Source: CAD feature listing. Evaluate the final solid. Frame: model axes, mm. A direction names the side the tool comes from. Give positions to 0.01 mm unless a question says otherwise; leave off trailing zeros. Order: outer loops, then holes, each group sorted by start corner. A loop starts at its lowest first (then second) coordinate and runs counter-clockwise, first axis right, second up. Notation, with made-up numbers: M 10,-26.75 L 31,-26.75 A15 ccw 31,-0.75 Z; hole C -28.5,89 d3. An arc over 180 degrees is marked long. Answer as a JSON object with one key per item and string values. Group by question number.
1. Section query D-D (y = 0.35). Count the separate pieces of the cut face and the enclosed holes in it, plus the area to 3 significant figures.
2. Section query C-C (z = 5.5). Output: boundary loops of the cut face in (x, y), plus the area to 3 significant figures.
3. Material intervals for L1, parallel to X at y = 1.4, z = 5.5; L2, parallel to X at y = 0.85, z = 5; L3, parallel to X at y = 1.65, z = 3.5, sorted ascending. Write a range as [from, to].
4. Set-up query: faces 4 (the flat face through (-17.19, 0.99, -13.73)), 5 (the cylindrical face through (-11.869, 0.986, 14.837)). Return all of +Z, -Z, +X, -X, +Y, -Y with unobstructed straight access to the full face (end or side cutting, diameter ignored); none if empty.
5. Section query A-A (x = 0). Output: boundary loops of the cut face in (y, z).
6. Section query B-B (z = 0). Output: boundary loops of the cut face in (x, y).
7. Pull-direction query (Z, two-part tool) for faces 1 (the flat face through (-17.214, 0.986, 13.699)), 2 (the cylindrical face through (-3.905, 0.986, -0.867)), 3 (the flat face through (0, 1, -22)); classes: +Z half, -Z half, draft (parallel to the pull), parting line (faces both ways), or undercut.
from build123d import *

# Parameters (mm, degrees)
SKETCH1_R           = 4
SKETCH1_R_2         = 1.5
BOSS_EXTRUDE1_DEPTH = 2


with BuildPart() as part:
    # Sketch1 → Boss-Extrude1 (new body)
    with BuildSketch(Plane(origin=(0, 0, 0), x_dir=(1, 0, 0), z_dir=(0, 1, 0))):
        with BuildLine():
            Line((0, 22), (-1.6, 22))
            add(Edge.make_bspline(
                [(-1.6, 22), (-2.318149564, 20.509493388), (-2.205951168, 18.871507079)],
                knots=[0, 0, 0, 1, 1, 1], degree=2))
            ThreePointArc((-2.205951168, 18.871507079), (-4.227897745, 18.523630331), (-6.200546728, 17.95976671))
            add(Edge.make_bspline(
                [(-8.103892072, 20.515529076), (-6.785743067, 19.501097309), (-6.200546728, 17.95976671)],
                knots=[0, 0, 0, 1, 1, 1], degree=2))
            Line((-8.103892072, 20.515529076), (-9.545442261, 19.821315094))
            Line((-9.545442261, 19.821315094), (-10.986992449, 19.127101111))
            add(Edge.make_bspline(
                [(-10.986992449, 19.127101111), (-10.987316267, 17.472607638), (-10.175533381, 16.045514028)],
                knots=[0, 0, 0, 1, 1, 1], degree=2))
            ThreePointArc((-10.175533381, 16.045514028), (-11.846306235, 14.854798167), (-13.3789503, 13.490874281))
            add(Edge.make_bspline(
                [(-16.202708931, 14.967706013), (-14.574952266, 14.62565799), (-13.3789503, 13.490874281)],
                knots=[0, 0, 0, 1, 1, 1], degree=2))
            Line((-16.202708931, 14.967706013), (-17.200292614, 13.716775641))
            Line((-17.200292614, 13.716775641), (-18.197876297, 12.465845269))
            add(Edge.make_bspline(
                [(-18.197876297, 12.465845269), (-17.480310233, 10.975057658), (-16.129726413, 10.041510138)],
                knots=[0, 0, 0, 1, 1, 1], degree=2))
            ThreePointArc((-16.129726413, 10.041510138), (-17.11840849, 8.243791043), (-17.907488682, 6.349948747))
            add(Edge.make_bspline(
                [(-21.092380574, 6.455345207), (-19.477413419, 6.853427735), (-17.907488682, 6.349948747)],
                knots=[0, 0, 0, 1, 1, 1], degree=2))
            Line((-21.092380574, 6.455345207), (-21.448414068, 4.895460547))
            Line((-21.448414068, 4.895460547), (-21.804447562, 3.335575888))
            add(Edge.make_bspline(
                [(-21.804447562, 3.335575888), (-20.511114375, 2.303762909), (-18.889229311, 2.048662014)],
                knots=[0, 0, 0, 1, 1, 1], degree=2))
            ThreePointArc((-18.889229311, 2.048662014), (-19, 0), (-18.889229311, -2.048662014))
            add(Edge.make_bspline(
                [(-21.804447562, -3.335575888), (-20.522133969, -2.276207935), (-18.889229311, -2.048662014)],
                knots=[0, 0, 0, 1, 1, 1], degree=2))
            Line((-21.804447562, -3.335575888), (-21.448414068, -4.895460547))
            Line((-21.448414068, -4.895460547), (-21.092380574, -6.455345207))
            add(Edge.make_bspline(
                [(-21.092380574, -6.455345207), (-19.479440763, -6.823820339), (-17.907488682, -6.349948747)],
                knots=[0, 0, 0, 1, 1, 1], degree=2))
            ThreePointArc((-17.907488682, -6.349948747), (-17.11840849, -8.243791043), (-16.129726413, -10.041510138))
            add(Edge.make_bspline(
                [(-18.197876297, -12.465845269), (-17.502194199, -10.955012707), (-16.129726413, -10.041510138)],
                knots=[0, 0, 0, 1, 1, 1], degree=2))
            Line((-18.197876297, -12.465845269), (-17.200292614, -13.716775641))
            Line((-17.200292614, -13.716775641), (-16.202708931, -14.967706013))
            add(Edge.make_bspline(
                [(-16.202708931, -14.967706013), (-14.589625008, -14.599862279), (-13.3789503, -13.490874281)],
                knots=[0, 0, 0, 1, 1, 1], degree=2))
            ThreePointArc((-13.3789503, -13.490874281), (-11.846306235, -14.854798167), (-10.175533381, -16.045514028))
            add(Edge.make_bspline(
                [(-10.986992449, -19.127101111), (-11.015730218, -17.464042859), (-10.175533381, -16.045514028)],
                knots=[0, 0, 0, 1, 1, 1], degree=2))
            Line((-10.986992449, -19.127101111), (-9.545442261, -19.821315094))
            Line((-9.545442261, -19.821315094), (-8.103892072, -20.515529076))
            add(Edge.make_bspline(
                [(-8.103892072, -20.515529076), (-6.81015509, -19.48422244), (-6.200546728, -17.95976671)],
                knots=[0, 0, 0, 1, 1, 1], degree=2))
            ThreePointArc((-6.200546728, -17.95976671), (-4.227897745, -18.523630331), (-2.205951168, -18.871507079))
            add(Edge.make_bspline(
                [(-1.6, -22), (-2.347465768, -20.514105139), (-2.205951168, -18.871507079)],
                knots=[0, 0, 0, 1, 1, 1], degree=2))
            Line((-1.6, -22), (0, -22))
            Line((0, -22), (1.6, -22))
            add(Edge.make_bspline(
                [(1.6, -22), (2.318149564, -20.509493388), (2.205951168, -18.871507079)],
                knots=[0, 0, 0, 1, 1, 1], degree=2))
            ThreePointArc((2.205951168, -18.871507079), (4.227897745, -18.523630331), (6.200546728, -17.95976671))
            add(Edge.make_bspline(
                [(8.103892072, -20.515529076), (6.785743067, -19.501097309), (6.200546728, -17.95976671)],
                knots=[0, 0, 0, 1, 1, 1], degree=2))
            Line((8.103892072, -20.515529076), (9.545442261, -19.821315094))
            Line((9.545442261, -19.821315094), (10.986992449, -19.127101111))
            add(Edge.make_bspline(
                [(10.986992449, -19.127101111), (10.987316267, -17.472607638), (10.175533381, -16.045514028)],
                knots=[0, 0, 0, 1, 1, 1], degree=2))
            ThreePointArc((10.175533381, -16.045514028), (11.846306235, -14.854798167), (13.3789503, -13.490874281))
            add(Edge.make_bspline(
                [(16.202708931, -14.967706013), (14.574952266, -14.62565799), (13.3789503, -13.490874281)],
                knots=[0, 0, 0, 1, 1, 1], degree=2))
            Line((16.202708931, -14.967706013), (17.200292614, -13.716775641))
            Line((17.200292614, -13.716775641), (18.197876297, -12.465845269))
            add(Edge.make_bspline(
                [(18.197876297, -12.465845269), (17.480310233, -10.975057658), (16.129726413, -10.041510138)],
                knots=[0, 0, 0, 1, 1, 1], degree=2))
            ThreePointArc((16.129726413, -10.041510138), (17.11840849, -8.243791043), (17.907488682, -6.349948747))
            add(Edge.make_bspline(
                [(21.092380574, -6.455345207), (19.477413419, -6.853427735), (17.907488682, -6.349948747)],
                knots=[0, 0, 0, 1, 1, 1], degree=2))
            Line((21.092380574, -6.455345207), (21.448414068, -4.895460547))
            Line((21.448414068, -4.895460547), (21.804447562, -3.335575888))
            add(Edge.make_bspline(
                [(21.804447562, -3.335575888), (20.511114375, -2.303762909), (18.889229311, -2.048662014)],
                knots=[0, 0, 0, 1, 1, 1], degree=2))
            ThreePointArc((18.889229311, -2.048662014), (19, 0), (18.889229311, 2.048662014))
            add(Edge.make_bspline(
                [(21.804447562, 3.335575888), (20.522133969, 2.276207935), (18.889229311, 2.048662014)],
                knots=[0, 0, 0, 1, 1, 1], degree=2))
            Line((21.804447562, 3.335575888), (21.448414068, 4.895460547))
            Line((21.448414068, 4.895460547), (21.092380574, 6.455345207))
            add(Edge.make_bspline(
                [(21.092380574, 6.455345207), (19.479440763, 6.823820339), (17.907488682, 6.349948747)],
                knots=[0, 0, 0, 1, 1, 1], degree=2))
            ThreePointArc((17.907488682, 6.349948747), (17.11840849, 8.243791043), (16.129726413, 10.041510138))
            add(Edge.make_bspline(
                [(18.197876297, 12.465845269), (17.502194199, 10.955012707), (16.129726413, 10.041510138)],
                knots=[0, 0, 0, 1, 1, 1], degree=2))
            Line((18.197876297, 12.465845269), (17.200292614, 13.716775641))
            Line((17.200292614, 13.716775641), (16.202708931, 14.967706013))
            add(Edge.make_bspline(
                [(16.202708931, 14.967706013), (14.589625008, 14.599862279), (13.3789503, 13.490874281)],
                knots=[0, 0, 0, 1, 1, 1], degree=2))
            ThreePointArc((13.3789503, 13.490874281), (11.846306235, 14.854798167), (10.175533381, 16.045514028))
            add(Edge.make_bspline(
                [(10.986992449, 19.127101111), (11.015730218, 17.464042859), (10.175533381, 16.045514028)],
                knots=[0, 0, 0, 1, 1, 1], degree=2))
            Line((10.986992449, 19.127101111), (9.545442261, 19.821315094))
            Line((9.545442261, 19.821315094), (8.103892072, 20.515529076))
            add(Edge.make_bspline(
                [(8.103892072, 20.515529076), (6.81015509, 19.48422244), (6.200546728, 17.95976671)],
                knots=[0, 0, 0, 1, 1, 1], degree=2))
            ThreePointArc((6.200546728, 17.95976671), (4.227897745, 18.523630331), (2.205951168, 18.871507079))
            add(Edge.make_bspline(
                [(1.6, 22), (2.347465768, 20.514105139), (2.205951168, 18.871507079)],
                knots=[0, 0, 0, 1, 1, 1], degree=2))
            Line((1.6, 22), (0, 22))
        make_face()
        with Locations(Location((0, 0, 0), (0, 0, 270))):
            Circle(SKETCH1_R, mode=Mode.SUBTRACT)
        with Locations(Location((0, 11, 0), (0, 0, 270))):
            Circle(SKETCH1_R_2, mode=Mode.SUBTRACT)
        with Locations(Location((9.526279442, -5.5, 0), (0, 0, 270))):
            Circle(SKETCH1_R_2, mode=Mode.SUBTRACT)
        with Locations(Location((-9.526279442, -5.5, 0), (0, 0, 270))):
            Circle(SKETCH1_R_2, mode=Mode.SUBTRACT)
    extrude(amount=BOSS_EXTRUDE1_DEPTH)


solid = part.part
Answer sheet:
{
 "1": {"separate pieces": "1", "enclosed holes": "4", "area": "1,240 mm^2"},
 "2": {"outline": "M -21.31,0 L -11.03,0 L -11.03,2 L -21.31,2 Z; M -8.03,0 L 8.03,0 L 8.03,2 L -8.03,2 Z; M 11.03,0 L 21.31,0 L 21.31,2 L 11.03,2 Z", "area": "73.2 mm^2"},
 "3": {"L1": "[-21.31, -11.03], [-8.03, 8.03], [11.03, 21.31]", "L2": "[-21.42, -10.94], [-8.11, 8.11], [10.94, 21.42]", "L3": "[-21.77, -1.94], [1.94, 21.77]"},
 "4": {"face 4": "-Z, -X, +Y, -Y", "face 5": "+Y, -Y"},
 "5": {"outline": "M 0,-22 L 2,-22 L 2,-12.5 L 0,-12.5 Z; M 0,-9.5 L 2,-9.5 L 2,-4 L 0,-4 Z; M 0,4 L 2,4 L 2,22 L 0,22 Z"},
 "6": {"outline": "M -19,0 L -4,0 L -4,2 L -19,2 Z; M 4,0 L 19,0 L 19,2 L 4,2 Z"},
 "7": {"face 1": "+Z half", "face 2": "undercut", "face 3": "-Z half"}
}
